Source: CAD feature listing. Evaluate the final solid. Frame: model axes, mm. Face numbers are marked on the shaded views. A direction names the side the tool comes from. Give positions to 0.01 mm unless a question says otherwise; leave off trailing zeros. Loops run counter-clockwise (first coordinate to the right, second up) from the corner with the lowest first, then second, coordinate; pieces in that order, holes last. Notation, with made-up numbers: (-32.5, -24) -> (-2.5, -24) arc R28 ccw to (-2.5, 3) -> close; hole circle Ø8 at (44, 48). An arc over 180 degrees is marked (long way). Return JSON: item names as keys, results as strings. Group by question number.
(1) Cut plane A-A on x = 21.5. Return loops of the section in (y, z).
(2) Draft query along X for the marked faces 6, 7, 8 and 9. Return one class per face: released by +X, released by -X, zero draft, split by the parting line, or undercut.
(3) Pin query (flat end, axial travel): pin 1 (1.5 mm diameter, centred on x = 12, y = -1.5, fed in from -Z); pin 2 (2 mm diameter, centred on y = -4.5, z = 16.5, fed in from -X); pin 3 (4 mm diameter, centred on y = -5, z = 14.5, fed in from +X); pin 4 (2 mm diameter, centred on y = -4.5, z = 7, fed in from -X). Return the tip coordinate at first contact, or that it passes through.
(4) Ray query, line 1 (Z direction, x = 29, y = -4.25); line 2 (Z direction, x = 9, y = -6.5); line 3 (X direction, y = -1.5, z = 17.75). Return the intervals inside material, ascending. Write a range as from..to.
(5) Cut plane D-D on x = 9. Return loops of the section in (y, z).
(6) Access query for the marked faces 1, 2, 3, 4 and 5. Directions: +Z, -Z, +X, -X, +Y, -Y. A direction counts if a zero-diameter tool reaches every point of the face in a straight line with its end or side. Return the directions, or none.
(7) Cut plane C-C on z = 16.75. Return loops of the section in (x, y).
(8) Cut plane B-B on y = -2.5. Return loops of the section in (x, z).
```python
from build123d import *

# Parameters (mm, degrees)
F1_DEPTH = 9
F2_W     = 11
F2_H     = 7
F3_DEPTH = 0.5


with BuildPart() as f1:
    # F0 (on Front) → F1 (new body)
    with BuildSketch(Plane.XZ):
        with BuildLine():
            Line((0, 1), (0, 0))
            Line((0, 0), (35, 0))
            ThreePointArc((35, 0), (44.75, 9.75), (35, 19.499999))
            Line((35, 19.499999), (12.5, 19.499999))
            ThreePointArc((12.5, 19.499999), (9, 15.999999), (5.5, 19.499999))
            Line((5.5, 19.499999), (0, 19.499999))
            Line((0, 19.499999), (0, 18.5))
            Line((0, 18.5), (4.612518, 18.5))
            ThreePointArc((4.612518, 18.5), (9, 15), (13.387482, 18.5))
            Line((13.387482, 18.5), (35, 18.5))
            ThreePointArc((35, 18.5), (43.75, 9.75), (35, 1))
            Line((35, 1), (0, 1))
        make_face()
    extrude(amount=F1_DEPTH)

    # F2 (on face) → F3 (cut)
    with BuildSketch(Plane(origin=(0, 0, 0), x_dir=(1, 0, 0), z_dir=(0, 0, -1))):
        with Locations((8.5, 4.5)):
            Rectangle(F2_W, F2_H)
    extrude(amount=-F3_DEPTH, mode=Mode.SUBTRACT)


solid = f1.part
```
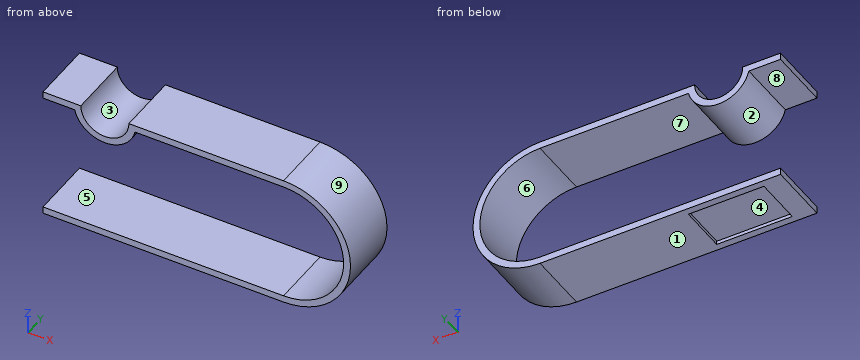
Answers:
{
 "1": {"outline": "(-9, 0) -> (0, 0) -> (0, 1) -> (-9, 1) -> close; (-9, 18.5) -> (0, 18.5) -> (0, 19.5) -> (-9, 19.5) -> close"},
 "2": {"face 6": "undercut", "face 7": "undercut", "face 8": "zero draft", "face 9": "released by +X"},
 "3": {"pin 1": "z = 0", "pin 2": "x = 4.97", "pin 3": "x = 44.35", "pin 4": "x = 42.91"},
 "4": {"line 1": "0..1, 18.5..19.5", "line 2": "0.5..1, 15..16", "line 3": "4.85..5.97, 12.03..13.15, 38.54..40.57"},
 "5": {"outline": "(-9, 0) -> (-8, 0) -> (-8, 0.5) -> (-1, 0.5) -> (-1, 0) -> (0, 0) -> (0, 1) -> (-9, 1) -> close; (-9, 15) -> (0, 15) -> (0, 16) -> (-9, 16) -> close"},
 "6": {"face 1": "-Z, +X, -X, +Y, -Y", "face 2": "+Y, -Y", "face 3": "+Z, +Y, -Y", "face 4": "-Z", "face 5": "-X, +Y, -Y"},
 "7": {"outline": "(5.44, -9) -> (6.83, -9) -> (6.83, 0) -> (5.44, 0) -> close; (11.17, -9) -> (12.56, -9) -> (12.56, 0) -> (11.17, 0) -> close; (40.25, -9) -> (41.79, -9) -> (41.79, 0) -> (40.25, 0) -> close"},
 "8": {"outline": "(0, 0) -> (3, 0) -> (3, 0.5) -> (14, 0.5) -> (14, 0) -> (35, 0) arc R9.75 ccw to (35, 19.5) -> (12.5, 19.5) arc R3.5 cw to (5.5, 19.5) -> (0, 19.5) -> (0, 18.5) -> (4.61, 18.5) arc R4.5 ccw to (13.39, 18.5) -> (35, 18.5) arc R8.75 cw to (35, 1) -> (0, 1) -> close"}
}
